Check sheet for the modelled part. Datum: model origin and axes. Units: mm. Give positions to 0.01 mm unless a question says otherwise; leave off trailing zeros. Loops run counter-clockwise (first coordinate to the right, second up) from the corner with the lowest first, then second, coordinate; pieces in that order, holes last. Notation, with made-up numbers: (24, -15) -> (43, -15) arc R19 ccw to (43, -9) -> close; hole circle Ø2 at (-29.5, 81). An arc over 180 degrees is marked (long way). Answer as CSV lines item,"result". Start each with the question number.
(1) Section check C-C on z = 25.5. State how many separate pieces and enclosed holes the cut face has, plus the area to 3 significant figures.
(2) Section check D-D on y = 8.5. Enter the section's corners in (x, z), plus the area to 3 significant figures.
(3) Section check A-A on x = -127. Enter the section's corners in (y, z).
(4) Material ranges on line 1 (X direction, y = 45, z = 30); line 2 (Z direction, x = -103, y = -126), recorded low to high. Write a range as from..to.
from build123d import *

# Parameters (mm, degrees)
F0_W     = 571.5
F0_H     = 571.5
F1_DEPTH = 38.1
F2_W     = 196.85
F2_H     = 25.4
F3_DEPTH = 571.501
F4_W     = 520.7
F4_H     = 25.4
F5_DEPTH = 571.501
F6_W     = 25.4
F6_H     = 127
F7_DEPTH = 38.1


with BuildPart() as f1:
    # F0 (on Top) → F1 (new body)
    with BuildSketch(Plane.XY):
        Rectangle(F0_W, F0_H)
    extrude(amount=F1_DEPTH)

    # F2 (on face) → F3 (cut, through all)
    with BuildSketch(Plane.XZ.offset(285.75)):
        with Locations((-161.925, 19.05)):
            Rectangle(F2_W, F2_H)
        with Locations((161.925, 19.05)):
            Rectangle(F2_W, F2_H)
    extrude(amount=-F3_DEPTH, mode=Mode.SUBTRACT)

    # F4 (on face) → F5 (cut, through all)
    with BuildSketch(Plane(origin=(-285.75, 0, 0), x_dir=(0, -1, 0), z_dir=(-1, 0, 0))):
        with Locations((0, 19.05)):
            Rectangle(F4_W, F4_H)
    extrude(amount=-F5_DEPTH, mode=Mode.SUBTRACT)

    # F6 (on face) → F7 (join)
    with BuildSketch(Plane.XY.offset(38.1)):
        with Locations((-273.05, 0)):
            Rectangle(F6_W, F6_H)
        with Locations((273.05, 0)):
            Rectangle(F6_W, F6_H)
    extrude(amount=-F7_DEPTH)


solid = f1.part
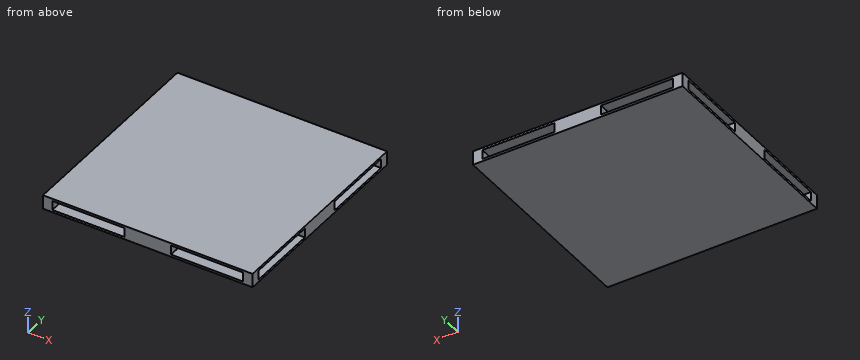
Working result:
1,separate pieces,"8"
1,enclosed holes,"0"
1,area,"15,500 mm^2"
2,outline,"(-285.75, 0) -> (285.75, 0) -> (285.75, 38.1) -> (-285.75, 38.1) -> close; hole (-260.35, 6.35) -> (260.35, 6.35) -> (260.35, 31.75) -> (-260.35, 31.75) -> close"
2,area,"8,550 mm^2"
3,outline,"(-285.75, 0) -> (285.75, 0) -> (285.75, 6.35) -> (-285.75, 6.35) -> close; (-285.75, 31.75) -> (285.75, 31.75) -> (285.75, 38.1) -> (-285.75, 38.1) -> close"
4,line 1,"x = -285.75..-260.35, 260.35..285.75"
4,line 2,"z = 0..6.35, 31.75..38.1"
